Design review of the part built by this model. Coordinates are the model's own, in mm. Face numbers are marked on the shaded views. A direction names the side the tool comes from. Round coordinates to 2 decimals unless told otherwise and drop trailing zeros. Order: outer loops, then holes, each group sorted by start corner. A loop starts at its lowest first (then second) coordinate and runs counter-clockwise, first axis right, second up. Notation, with made-up numbers: (83, -34.5) - (91, -34.5) arc R20 ccw to (91, -9.5) - close; hole circle Ø4 at (5.25, -20). An arc over 180 degrees is marked (long way). Write item = value, one per line.
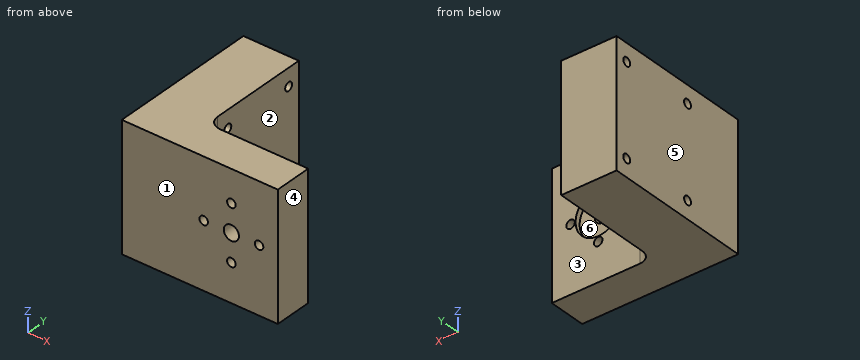
from build123d import *

# Parameters (mm, degrees)
BOSS_EXTRUDE1_DEPTH = 50
FILLET1_R           = 5
SKETCH2_R           = 1.7
CUT_EXTRUDE1_DEPTH  = 50
SKETCH3_R           = 9
CUT_EXTRUDE4_DEPTH  = 2
SKETCH4_R           = 3
CUT_EXTRUDE5_DEPTH  = 15
SKETCH5_R           = 1.7
CUT_EXTRUDE6_DEPTH  = 81.131020262


with BuildPart() as part:
    # Sketch1 → Boss-Extrude1 (new body)
    with BuildSketch(Plane.XY):
        Polygon((-43.542857143, 31.8), (-43.542857143, -28.2), (18.457142857, -28.2), (18.457142857, -13.2), (-21.542857143, -13.2), (-21.542857143, 31.8), align=None)
    extrude(amount=BOSS_EXTRUDE1_DEPTH)

    # Fillet1
    fillet1_edges = [part.edges().sort_by_distance(p)[0] for p in [
        (-21.542857143, -13.2, 25),
    ]]
    fillet(fillet1_edges, radius=FILLET1_R)

    # Sketch2 → Cut-Extrude1 (cut)
    with BuildSketch(Plane(origin=(-21.542857143, 0, 0), x_dir=(0, 0, -1), z_dir=(1, 0, 0))):
        with Locations(Location((-43, 26.8, 0), (0, 0, 90))):
            Circle(SKETCH2_R)
        with Locations(Location((-7, 26.8, 0), (0, 0, 90))):
            Circle(SKETCH2_R)
        with Locations(Location((-7, -3.2, 0), (0, 0, 90))):
            Circle(SKETCH2_R)
        with Locations(Location((-43, -3.2, 0), (0, 0, 90))):
            Circle(SKETCH2_R)
    extrude(amount=-CUT_EXTRUDE1_DEPTH, mode=Mode.SUBTRACT)

    # Sketch3 → Cut-Extrude4 (cut)
    with BuildSketch(Plane(origin=(0, -13.2, 0), x_dir=(1, 0, 0), z_dir=(0, 1, 0))):
        with Locations(Location((0, -26.167935948, 0), (0, 0, 180))):
            Circle(SKETCH3_R)
    extrude(amount=-CUT_EXTRUDE4_DEPTH, mode=Mode.SUBTRACT)

    # Sketch4 → Cut-Extrude5 (cut)
    with BuildSketch(Plane(origin=(0, -13.2, 0), x_dir=(1, 0, 0), z_dir=(0, 1, 0))):
        with Locations(Location((0, -26.167935948, 0), (0, 0, 180))):
            Circle(SKETCH4_R)
    extrude(amount=-CUT_EXTRUDE5_DEPTH, mode=Mode.SUBTRACT)

    # Sketch5 → Cut-Extrude6 (cut, through all)
    with BuildSketch(Plane(origin=(0, -13.2, 0), x_dir=(1, 0, 0), z_dir=(0, 1, 0))):
        with Locations(Location((-11, -26.167935948, 0), (0, 0, 180))):
            Circle(SKETCH5_R)
        with Locations(Location((0, -15.167935948, 0), (0, 0, 180))):
            Circle(SKETCH5_R)
        with Locations(Location((11, -26.167935948, 0), (0, 0, 180))):
            Circle(SKETCH5_R)
        with Locations(Location((0, -37.167935948, 0), (0, 0, 180))):
            Circle(SKETCH5_R)
    extrude(amount=-CUT_EXTRUDE6_DEPTH, mode=Mode.SUBTRACT)


solid = part.part
1) To check wall thickness, follow L1, parallel to Z at x = 0, y = -19.25; L2, parallel to Z at x = -30, y = -3.2; L3, parallel to X at y = 16, z = 47. State the ranges of each line that lie inside material, in increasing order. Write a range as from..to.
Findings:
L1 = 0..13.47, 16.87..23.17, 29.17..35.47, 38.87..50
L2 = 0..5.3, 8.7..41.3, 44.7..50
L3 = -43.54..-21.54
2) We need section D-D on y = -3.2. Write out the cut boundary in (x, z), and give its area (3 significant figures).
Findings:
outline = (-43.54, 0) - (-21.54, 0) - (-21.54, 5.3) - (-43.54, 5.3) - close; (-43.54, 8.7) - (-21.54, 8.7) - (-21.54, 41.3) - (-43.54, 41.3) - close; (-43.54, 44.7) - (-21.54, 44.7) - (-21.54, 50) - (-43.54, 50) - close
area = 950 mm^2
3) We need section C-C on x = 0. Write out the cut boundary in (y, z).
Findings:
outline = (-28.2, 0) - (-13.2, 0) - (-13.2, 13.47) - (-28.2, 13.47) - close; (-28.2, 16.87) - (-13.2, 16.87) - (-13.2, 17.17) - (-15.2, 17.17) - (-15.2, 23.17) - (-28.2, 23.17) - close; (-28.2, 29.17) - (-15.2, 29.17) - (-15.2, 35.17) - (-13.2, 35.17) - (-13.2, 35.47) - (-28.2, 35.47) - close; (-28.2, 38.87) - (-13.2, 38.87) - (-13.2, 50) - (-28.2, 50) - close
4) We need section B-B on z = 7. Write out the cut boundary in (x, y), and give its area (3 significant figures).
Findings:
outline = (-43.54, -28.2) - (18.46, -28.2) - (18.46, -13.2) - (-16.54, -13.2) arc R5 cw to (-21.54, -8.2) - (-21.54, -4.9) - (-43.54, -4.9) - close; (-43.54, -1.5) - (-21.54, -1.5) - (-21.54, 25.1) - (-43.54, 25.1) - close; (-43.54, 28.5) - (-21.54, 28.5) - (-21.54, 31.8) - (-43.54, 31.8) - close
area = 1,780 mm^2
5) The part is to be moulded in two halves that separate along X. For the marked faces 3, 4, 5 and 6, say which applies: released by +X, released by -X, zero draft, split by the parting line, or undercut.
Findings:
face_3 = zero draft
face_4 = released by +X
face_5 = released by -X
face_6 = undercut
6) Clearance check with flat-ended pins moving along their axes: pin 1 Ø17.5 at (x, z) = (1.5, 26) entering from +Y; pin 2 Ø3 at (y, z) = (-3.2, 43) entering from +X; pin 3 Ø3 at (y, z) = (1.5, 41) entering from +X; pin 4 Ø3 at (x, z) = (2.5, 22) entering from +Y. State where each tip first meets the part, or that it passes through.
Findings:
pin_1 = -13.2
pin_2 = through
pin_3 = -21.54
pin_4 = -15.2
7) For the marked faces 1 and 2, list the 3-axis set-ups (+Z, -Z, +X, -X, +Y, -Y) from which the entire face can be reached by the end or side of a thin tool; tool diameter is ignored.
Findings:
face_1 = +Z, -Z, +X, -X, -Y
face_2 = +Z, -Z, +X, +Y
8) We need section A-A on x = 11. Write out the cut boundary in (y, z), and give its area (3 significant figures).
Findings:
outline = (-28.2, 0) - (-13.2, 0) - (-13.2, 24.47) - (-28.2, 24.47) - close; (-28.2, 27.87) - (-13.2, 27.87) - (-13.2, 50) - (-28.2, 50) - close
area = 699 mm^2
